Check sheet for the modelled part. Datum: model origin and axes. Units: mm. Coordinates: 2 decimals unless noted, no trailing zeros. Loops run counter-clockwise (first coordinate to the right, second up) from the corner with the lowest first, then second, coordinate; pieces in that order, holes last. Notation, with made-up numbers: M 88,-25.5 L 127,-25.5 A18 cw 127,-7.5 Z; hole C 61,87.25 d5. An arc over 180 degrees is marked long. Use CSV: the item, a comma, the result in double quotes. Start each with the question number.
(1) Section check A-A on y = 3.95. Give the number of separate pieces and of enclosed holes in the cut face, and give its area (3 significant figures).
(2) Go/stop test with flat-tipped pins: pin 1 Ø3 at (y, z) = (3.5, -1.5) entering from +X; pin 2 Ø2 at (y, z) = (2, -36.5) entering from -X; pin 3 Ø0.6 at (y, z) = (2.5, -25) entering from -X. Record where each tip stops, or that it passes through.
(3) Scan lines: line 1 (X direction, y = 4.05, z = -10); line 2 (Z direction, x = 65, y = 4.25); line 3 (X direction, y = 2.05, z = -49). Record each from-to range of solid material in increasing order.
(4) Section check B-B on x = -31.5. Record the cut outline in (y, z), and give its area (3 significant figures).
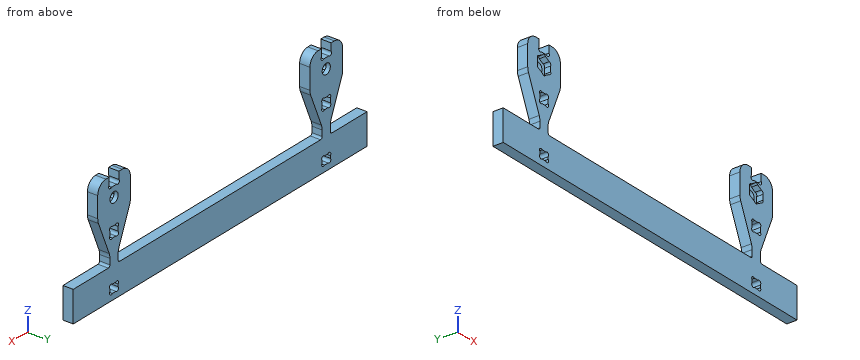
from build123d import *

# Parameters (mm, degrees)
SKETCH_1_R           = 2.5
EXTRUDE_1_DEPTH      = 5
FILLET_1_R           = 5
SKETCH_6_W           = 6
SKETCH_6_H           = 5
CUT_EXTRUDE_5_DEPTH  = 10
SKETCH_7_R           = 1
CUT_EXTRUDE_6_DEPTH  = 10
SKETCH_8_W           = 7.5
SKETCH_8_H           = 5
CUT_EXTRUDE_7_DEPTH  = 10
FILLET_2_R           = 1
CUT_EXTRUDE_9_DEPTH  = 10
FILLET_3_R           = 6
SKETCH_12_W          = 5
SKETCH_12_H          = 4
SKETCH_12_H_2        = 5
CUT_EXTRUDE_10_DEPTH = 5
CUT_EXTRUDE_12_DEPTH = 3
SKETCH_15_R          = 1
CUT_EXTRUDE_13_DEPTH = 3
SKETCH_16_R          = 1
SKETCH_16_R_2        = 1.016973241
CUT_EXTRUDE_14_DEPTH = 10


with BuildPart() as part:
    # 스케치1 → 보스-돌출1 (new body)
    with BuildSketch(Plane(origin=(0, 0, 0), x_dir=(1, 0, 0), z_dir=(0, 1, 0))):
        Polygon((-90, 54.2), (90, 54.2), (90, 39.2), (75, 39.2), (75, 0), (55, 0), (55, 39.2), (-55, 39.2), (-55, 0), (-75, 0), (-75, 39.2), (-90, 39.2), align=None)
        with Locations(Location((65, 10, 0), (0, 0, 270))):
            Circle(SKETCH_1_R, mode=Mode.SUBTRACT)
        with Locations(Location((-65, 10, 0), (0, 0, 90))):
            Circle(SKETCH_1_R, mode=Mode.SUBTRACT)
    extrude(amount=EXTRUDE_1_DEPTH)

    # 필렛1
    fillet_1_edges = [part.edges().sort_by_distance(p)[0] for p in [
        (75, 2.5, 0),
        (55, 2.5, 0),
        (-55, 2.5, 0),
        (-75, 2.5, 0),
    ]]
    fillet(fillet_1_edges, radius=FILLET_1_R)

    # 스케치6 → 컷-돌출5 (cut)
    with BuildSketch(Plane.XZ):
        with Locations((65, -2.5)):
            Rectangle(SKETCH_6_W, SKETCH_6_H)
        with Locations((-65, -2.5)):
            Rectangle(SKETCH_6_W, SKETCH_6_H)
    extrude(amount=-CUT_EXTRUDE_5_DEPTH, mode=Mode.SUBTRACT)

    # 스케치7 → 컷-돌출6 (cut)
    with BuildSketch(Plane.XZ):
        with Locations((62.707106781, -4.292893219)):
            Circle(SKETCH_7_R)
        with Locations((67.292893219, -4.292893219)):
            Circle(SKETCH_7_R)
        with Locations((-67.292893219, -4.292893219)):
            Circle(SKETCH_7_R)
        with Locations((-62.707106781, -4.292893219)):
            Circle(SKETCH_7_R)
    extrude(amount=-CUT_EXTRUDE_6_DEPTH, mode=Mode.SUBTRACT)

    # 스케치8 → 컷-돌출7 (cut)
    with BuildSketch(Plane(origin=(0, 5, 0), x_dir=(1, 0, 0), z_dir=(0, 1, 0))):
        with Locations((71.25, 36.7)):
            Rectangle(SKETCH_8_W, SKETCH_8_H)
        with Locations((58.75, 36.7)):
            Rectangle(SKETCH_8_W, SKETCH_8_H)
        with Locations((-58.75, 36.7)):
            Rectangle(SKETCH_8_W, SKETCH_8_H)
        with Locations((-71.25, 36.7)):
            Rectangle(SKETCH_8_W, SKETCH_8_H)
    extrude(amount=-CUT_EXTRUDE_7_DEPTH, mode=Mode.SUBTRACT)

    # 필렛2
    fillet_2_edges = [part.edges().sort_by_distance(p)[0] for p in [
        (67.5, 2.5, -39.2),
        (62.5, 2.5, -39.2),
        (-62.5, 2.5, -39.2),
        (-67.5, 2.5, -39.2),
    ]]
    fillet(fillet_2_edges, radius=FILLET_2_R)

    # 스케치10 → 컷-돌출9 (cut)
    with BuildSketch(Plane(origin=(0, 5, 0), x_dir=(1, 0, 0), z_dir=(0, 1, 0))):
        Polygon((75, 34.2), (67.5, 34.2), (75, 16.2), align=None)
        Polygon((62.5, 34.2), (55, 34.2), (55, 16.2), align=None)
        Polygon((-75, 16.2), (-75, 34.2), (-67.5, 34.2), align=None)
        Polygon((-55, 16.2), (-55, 34.2), (-62.5, 34.2), align=None)
    extrude(amount=-CUT_EXTRUDE_9_DEPTH, mode=Mode.SUBTRACT)

    # 필렛3
    fillet_3_edges = [part.edges().sort_by_distance(p)[0] for p in [
        (67.5, 2.5, -34.2),
        (62.5, 2.5, -34.2),
        (-62.5, 2.5, -34.2),
        (-67.5, 2.5, -34.2),
        (75, 2.5, -16.2),
        (55, 2.5, -16.2),
        (-75, 2.5, -16.2),
        (-55, 2.5, -16.2),
    ]]
    fillet(fillet_3_edges, radius=FILLET_3_R)

    # 스케치12 → 컷-돌출10 (cut)
    with BuildSketch(Plane(origin=(0, 5, 0), x_dir=(1, 0, 0), z_dir=(0, 1, 0))):
        with Locations((65, 49.2)):
            Rectangle(SKETCH_12_W, SKETCH_12_H)
        with Locations((65, 24.7)):
            Rectangle(SKETCH_12_W, SKETCH_12_H_2)
        with Locations((-65, 24.7)):
            Rectangle(SKETCH_12_W, SKETCH_12_H_2)
        with Locations((-65, 49.2)):
            Rectangle(SKETCH_12_W, SKETCH_12_H)
    extrude(amount=-CUT_EXTRUDE_10_DEPTH, mode=Mode.SUBTRACT)

    # 스케치14 → 컷-돌출12 (cut)
    with BuildSketch(Plane(origin=(0, 0, 0), x_dir=(-1, 0, 0), z_dir=(0, -1, 0))):
        Polygon((-65, 14.618802154), (-69, 12.309401077), (-69, 7.690598923), (-65, 5.381197846), (-61, 7.690598923), (-61, 12.309401077), align=None)
        Polygon((65, 14.618802154), (61, 12.309401077), (61, 7.690598923), (65, 5.381197846), (69, 7.690598923), (69, 12.309401077), align=None)
    extrude(amount=-CUT_EXTRUDE_12_DEPTH, mode=Mode.SUBTRACT)

    # 스케치15 → 컷-돌출13 (cut)
    with BuildSketch(Plane.XZ):
        with Locations((65, -13.618802154)):
            Circle(SKETCH_15_R)
        with Locations((61.866025404, -11.809401077)):
            Circle(SKETCH_15_R)
        with Locations((61.866025404, -8.190598923)):
            Circle(SKETCH_15_R)
        with Locations((65, -6.381197846)):
            Circle(SKETCH_15_R)
        with Locations((68.133974596, -8.190598923)):
            Circle(SKETCH_15_R)
        with Locations((68.133974596, -11.809401077)):
            Circle(SKETCH_15_R)
        with Locations((-68.133974596, -11.809401077)):
            Circle(SKETCH_15_R)
        with Locations((-68.133974596, -8.190598923)):
            Circle(SKETCH_15_R)
        with Locations((-65, -6.381197846)):
            Circle(SKETCH_15_R)
        with Locations((-61.866025404, -8.190598923)):
            Circle(SKETCH_15_R)
        with Locations((-61.866025404, -11.809401077)):
            Circle(SKETCH_15_R)
        with Locations((-65, -13.618802154)):
            Circle(SKETCH_15_R)
    extrude(amount=-CUT_EXTRUDE_13_DEPTH, mode=Mode.SUBTRACT)

    # 스케치16 → 컷-돌출14 (cut)
    with BuildSketch(Plane.XZ):
        with Locations((66.792893219, -47.907106781)):
            Circle(SKETCH_16_R)
        with Locations((66.792893219, -50.492893219)):
            Circle(SKETCH_16_R)
        with Locations((63.207106781, -50.492893219)):
            Circle(SKETCH_16_R)
        with Locations((63.207106781, -47.907106781)):
            Circle(SKETCH_16_R)
        with Locations((66.780891325, -22.919108675)):
            Circle(SKETCH_16_R_2)
        with Locations((63.219108675, -22.919108675)):
            Circle(SKETCH_16_R_2)
        with Locations((63.219108675, -26.480891325)):
            Circle(SKETCH_16_R_2)
        with Locations((66.780891325, -26.480891325)):
            Circle(SKETCH_16_R_2)
        with Locations((-66.780891325, -26.480891325)):
            Circle(SKETCH_16_R_2)
        with Locations((-63.219108675, -26.480891325)):
            Circle(SKETCH_16_R_2)
        with Locations((-63.219108675, -22.919108675)):
            Circle(SKETCH_16_R_2)
        with Locations((-66.780891325, -22.919108675)):
            Circle(SKETCH_16_R_2)
        with Locations((-63.207106781, -47.907106781)):
            Circle(SKETCH_16_R)
        with Locations((-63.207106781, -50.492893219)):
            Circle(SKETCH_16_R)
        with Locations((-66.792893219, -50.492893219)):
            Circle(SKETCH_16_R)
        with Locations((-66.792893219, -47.907106781)):
            Circle(SKETCH_16_R)
    extrude(amount=-CUT_EXTRUDE_14_DEPTH, mode=Mode.SUBTRACT)


solid = part.part
Outcome:
1,separate pieces,"1"
1,enclosed holes,"6"
1,area,"3,630 mm²"
2,pin 1,"stops at x = 74.58"
2,pin 2,"stops at x = -67.5"
2,pin 3,"stops at x = -71.46"
3,line 1,"x = -75 to -67.5, -62.5 to -55, 55 to 62.5, 67.5 to 75"
3,line 2,"z = -54.2 to -51.2, -47.2 to -27.2, -22.2 to -12.5, -7.5 to -5"
3,line 3,"x = -90 to -67.5, -62.5 to 62.5, 67.5 to 90"
4,outline,"M 0,-54.2 L 5,-54.2 L 5,-39.2 L 0,-39.2 Z"
4,area,"75.0 mm²"
